Read the model definition and answer for the solid it produces. Units are mm, in the model's axes. Face numbers are marked on the shaded views. A direction names the side the tool comes from. Coordinates: 2 decimals unless noted, no trailing zeros. Order: outer loops, then holes, each group sorted by start corner. A loop starts at its lowest first (then second) coordinate and runs counter-clockwise, first axis right, second up. Notation, with made-up numbers: (24.25, 83.5) -> (64.25, 83.5) arc R27 ccw to (64.25, 119.5) -> close; hole circle Ø10 at (-7.5, 88.25). An arc over 180 degrees is marked (long way). Answer in a Markdown table with one row per item.
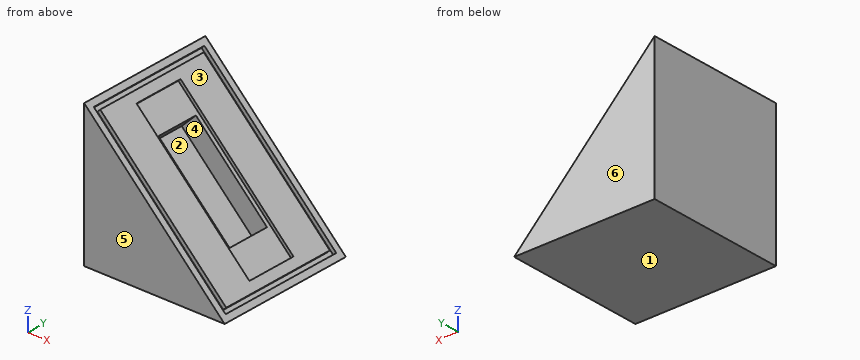
from build123d import *

# Parameters (mm, degrees)
SKETCH1_W           = 69.85
SKETCH1_H           = 69.85
BOSS_EXTRUDE1_DEPTH = 69.85
CUT_EXTRUDE2_DEPTH  = 100
SKETCH3_W           = 92.686817332
SKETCH3_H           = 63.754
SKETCH3_W_2         = 88.622817332
SKETCH3_H_2         = 59.69
CUT_EXTRUDE4_DEPTH  = 2.032
SKETCH4_W           = 79.375
SKETCH4_H           = 25.4
CUT_EXTRUDE5_DEPTH  = 1.6
SKETCH5_W           = 50
SKETCH5_H           = 21.59
CUT_EXTRUDE6_DEPTH  = 10


with BuildPart() as part:
    # Sketch1 → Boss-Extrude1 (new body)
    with BuildSketch(Plane(origin=(0, 0, 0), x_dir=(1, 0, 0), z_dir=(0, 1, 0))):
        with Locations((34.925, 34.925)):
            Rectangle(SKETCH1_W, SKETCH1_H)
    extrude(amount=BOSS_EXTRUDE1_DEPTH)

    # Sketch2 → Cut-Extrude2 (cut)
    with BuildSketch(Plane(origin=(0, 0, 0), x_dir=(0.707106781, 0, -0.707106781), z_dir=(0.707106781, 0, 0.707106781))):
        Polygon((98.782817332, 69.85), (98.782817332, 0), (49.391408666, 0), (0, 0), (0, 69.85), (49.391408666, 69.85), align=None)
    extrude(amount=CUT_EXTRUDE2_DEPTH, mode=Mode.SUBTRACT)

    # Sketch3 → Cut-Extrude4 (cut)
    with BuildSketch(Plane(origin=(0, 0, 0), x_dir=(0.707106781, 0, -0.707106781), z_dir=(0.707106781, 0, 0.707106781))):
        with Locations((49.391408666, 34.925)):
            Rectangle(SKETCH3_W, SKETCH3_H)
        with Locations((49.391408666, 34.925)):
            Rectangle(SKETCH3_W_2, SKETCH3_H_2, mode=Mode.SUBTRACT)
    extrude(amount=-CUT_EXTRUDE4_DEPTH, mode=Mode.SUBTRACT)

    # Sketch4 → Cut-Extrude5 (cut)
    with BuildSketch(Plane(origin=(0, 0, 0), x_dir=(0.707106781, 0, -0.707106781), z_dir=(0.707106781, 0, 0.707106781))):
        with Locations((49.391408666, 34.925)):
            Rectangle(SKETCH4_W, SKETCH4_H)
    extrude(amount=-CUT_EXTRUDE5_DEPTH, mode=Mode.SUBTRACT)

    # Sketch5 → Cut-Extrude6 (cut)
    with BuildSketch(Plane(origin=(-1.13137085, 0, -1.13137085), x_dir=(0.707106781, 0, -0.707106781), z_dir=(0.707106781, 0, 0.707106781))):
        with Locations((49.391408666, 34.925)):
            Rectangle(SKETCH5_W, SKETCH5_H)
    extrude(amount=-CUT_EXTRUDE6_DEPTH, mode=Mode.SUBTRACT)


solid = part.part
Q1. For the marked faces 1 and 2, determine the directions among +Z, -Z, +X, -X, +Y, -Y from which every point of the face is accessible in a straight line to the end or side of a thin tool.
Outcome:
| item | result |
|---|---|
| face 1 | -Z, +X, -X, +Y, -Y |
| face 2 | none |
Q2. For a pull along Y with two mould halves and no side action, classify the marked faces 3, 4, 5 and 6 as pulls with the +Y half, pulls with the -Y half, needs draft (parallel to the pull), parting line crosses it, or undercut.
Outcome:
| item | result |
|---|---|
| face 3 | needs draft |
| face 4 | undercut |
| face 5 | pulls with the -Y half |
| face 6 | pulls with the +Y half |
Q3. The part is cut by section A-A (y = 9.5). Write down the section's boundary in (x, z), then the cut area to 3 significant figures.
Outcome:
| item | result |
|---|---|
| outline | (0, -69.85) -> (69.85, -69.85) -> (67.69, -67.69) -> (66.26, -69.13) -> (64.82, -67.69) -> (66.26, -66.26) -> (3.59, -3.59) -> (2.16, -5.03) -> (0.72, -3.59) -> (2.16, -2.16) -> (0, 0) -> close |
| area | 2,430 mm² |
Q4. The part is cut by section B-B (z = -58). Write down the section's boundary in (x, y) (3 decimals).
Outcome:
| item | result |
|---|---|
| outline | (0, 0) -> (58, 0) -> (58, 3.048) -> (55.126, 3.048) -> (55.126, 5.08) -> (58, 5.08) -> (58, 22.225) -> (55.737, 22.225) -> (55.737, 47.625) -> (58, 47.625) -> (58, 64.77) -> (55.126, 64.77) -> (55.126, 66.802) -> (58, 66.802) -> (58, 69.85) -> (0, 69.85) -> close; hole (41.595, 24.13) -> (47.205, 24.13) -> (47.205, 45.72) -> (41.595, 45.72) -> close |
Q5. Given pin 1 (8 mm diameter, centred on y = 53, z = -39.5, fed in from -X); pin 2 (2 mm diameter, centred on x = 37.5, y = 45, fed in from +Z), each flat-ended and moving along its own axis, determine where each tip first touches the part or whether it passes through.
Outcome:
| item | result |
|---|---|
| pin 1 | x = 0 |
| pin 2 | z = -39.07 |
Q6. Consider line 1 (Y direction, x = 5.5, z = -6); line 2 (Y direction, x = 40, z = -43); line 3 (Z direction, x = 65.5, y = 13). Determine where each line is inside the solid, lowest interval first.
Outcome:
| item | result |
|---|---|
| line 1 | 0 to 3.05, 5.08 to 64.77, 66.8 to 69.85 |
| line 2 | 0 to 24.13, 45.72 to 69.85 |
| line 3 | -69.85 to -68.37, -67.02 to -65.5 |
Q7. The part is cut by section D-D (z = -33). Write down the section's boundary in (x, y) (3 decimals).
Outcome:
| item | result |
|---|---|
| outline | (0, 0) -> (33, 0) -> (33, 3.048) -> (30.126, 3.048) -> (30.126, 5.08) -> (33, 5.08) -> (33, 22.225) -> (30.737, 22.225) -> (30.737, 24.13) -> (16.595, 24.13) -> (16.595, 45.72) -> (30.737, 45.72) -> (30.737, 47.625) -> (33, 47.625) -> (33, 64.77) -> (30.126, 64.77) -> (30.126, 66.802) -> (33, 66.802) -> (33, 69.85) -> (0, 69.85) -> close |
Q8. The part is cut by section C-C (x = 46.5). Write down the section's boundary in (y, z) (3 decimals).
Outcome:
| item | result |
|---|---|
| outline | (0, -69.85) -> (69.85, -69.85) -> (69.85, -46.5) -> (66.802, -46.5) -> (66.802, -49.374) -> (64.77, -49.374) -> (64.77, -46.5) -> (47.625, -46.5) -> (47.625, -48.763) -> (45.72, -48.763) -> (45.72, -58.705) -> (24.13, -58.705) -> (24.13, -48.763) -> (22.225, -48.763) -> (22.225, -46.5) -> (5.08, -46.5) -> (5.08, -49.374) -> (3.048, -49.374) -> (3.048, -46.5) -> (0, -46.5) -> close |
